```python
from build123d import *

# Parameters (mm, degrees)
SKETCH2_W           = 2.5
SKETCH2_H           = 2.5
BOSS_EXTRUDE1_DEPTH = 39
SKETCH3_W           = 2.5
SKETCH3_H           = 1
BOSS_EXTRUDE2_DEPTH = 3
CUT_EXTRUDE1_DEPTH  = 2.5
FILLET1_R           = 1
BOSS_EXTRUDE3_DEPTH = 2.5
SKETCH8_W           = 2.5
SKETCH8_H           = 2
BOSS_EXTRUDE4_DEPTH = 4


with BuildPart() as part:
    # Sketch2 → Boss-Extrude1 (new body)
    with BuildSketch(Plane(origin=(0, 0, 0), x_dir=(1, 0, 0), z_dir=(0, 1, 0))):
        Rectangle(SKETCH2_W, SKETCH2_H)
    extrude(amount=BOSS_EXTRUDE1_DEPTH)

    # Sketch3 → Boss-Extrude2 (add)
    with BuildSketch(Plane.XY.offset(1.25)):
        with Locations((0, 0.5)):
            Rectangle(SKETCH3_W, SKETCH3_H)
    extrude(amount=BOSS_EXTRUDE2_DEPTH)

    # Sketch4 → Cut-Extrude1 (cut)
    with BuildSketch(Plane(origin=(1.25, 0, 0), x_dir=(0, 0, -1), z_dir=(1, 0, 0))):
        Polygon((-4.25, 0), (-4.25, 0.75), (1.25, 0), align=None)
    extrude(amount=-CUT_EXTRUDE1_DEPTH, mode=Mode.SUBTRACT)

    # Fillet1
    fillet1_edges = [part.edges().sort_by_distance(p)[0] for p in [
        (0, 0, -1.25),
    ]]
    fillet(fillet1_edges, radius=FILLET1_R)

    # Sketch6 → Boss-Extrude3 (add)
    with BuildSketch(Plane.XY.offset(1.25)):
        Polygon((1.25, 20.2), (1.25, 21.8), (3, 21.8), (3, 22.2), (4, 22.2), (4, 19.8), (3, 19.8), (3, 20.2), align=None)
    extrude(amount=-BOSS_EXTRUDE3_DEPTH)

    # Sketch8 → Boss-Extrude4 (add)
    with BuildSketch(Plane.XY.offset(1.25)):
        with Locations((0, 29.4)):
            Rectangle(SKETCH8_W, SKETCH8_H)
    extrude(amount=BOSS_EXTRUDE4_DEPTH)


solid = part.part
```
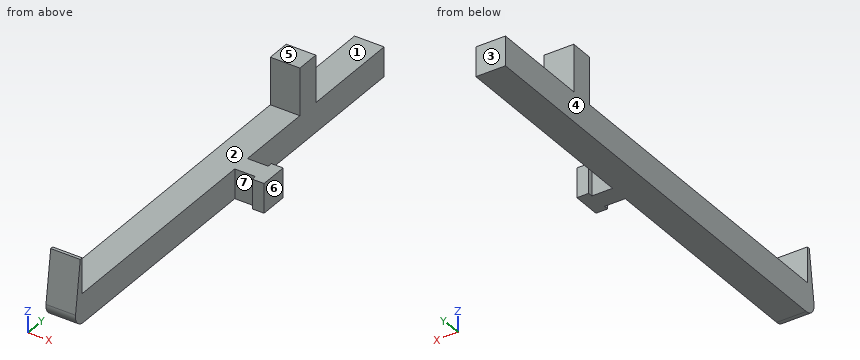
Check sheet for the modelled part. Datum: model origin and axes. Units: mm. Face numbers are marked on the shaded views. A direction names the side the tool comes from. Coordinates: 2 decimals unless noted, no trailing zeros. Write each loop counter-clockwise with the first axis right and the second up, starting at its lowest first coordinate (ties: lowest second). Pieces come first, ordered by that corner, then holes. Notation, with made-up numbers: M 88,41 L 112,41 A27 ccw 112,57 Z; hole C 49,-24 d2. An arc over 180 degrees is marked long. Write item = value, one per line. Start each with the question number.
1. Mould release check, pull along X, two halves, no side actions. Record for the marked faces 4, 5, 6 and 7: pulls with the +X half, pulls with the -X half, needs draft (parallel to the pull), parting line crosses it, or undercut.
2. Sectioned sample at D-D (x = 3.6). Record the cut outline in (y, z).
3. Sectioned sample at C-C (y = 30). Record the cut outline in (x, z).
4. Thickness scan on probe 1 along X at (y, z) = (19.5, 1); probe 2 along Y at (x, z) = (0.85, 4). Record the ranges inside material, lowest first.
5. Go/stop test with flat-tipped pins: pin 1 (2 mm diameter, centred on y = 24, z = 2, fed in from +X); pin 2 (0.8 mm diameter, centred on x = 3.5, z = 0, fed in from +Y); pin 3 (0.5 mm diameter, centred on x = 2, z = 0, fed in from -Y). Record where each tip stops, or that it passes through.
6. Sectioned sample at A-A (x = -0.1). Record the cut outline in (y, z), then the cut area to 3 significant figures.
7. Tool access check on the marked faces 1, 2 and 3. Record the directions out of +Z, -Z, +X, -X, +Y, -Y that give a thin tool (end or side, any length) a straight path to the whole face; none if there is none.
8. Sectioned sample at B-B (z = 0.5). Record the cut outline in (x, y), then the cut area to 3 significant figures.
The answers:
q1.face_4 = pulls with the -X half
q1.face_5 = needs draft
q1.face_6 = pulls with the +X half
q1.face_7 = undercut
q2.outline = M 19.8,-1.25 L 22.2,-1.25 L 22.2,1.25 L 19.8,1.25 Z
q3.outline = M -1.25,-1.25 L 1.25,-1.25 L 1.25,5.25 L -1.25,5.25 Z
q4.probe_1 = -1.25 to 1.25
q4.probe_2 = 0.72 to 1, 28.4 to 30.4
q5.pin_1 = 1.25
q5.pin_2 = 22.2
q5.pin_3 = 20.2
q6.outline = M 0.15,-0.11 A1 ccw 1.15,-1.25 L 39,-1.25 L 39,1.25 L 30.4,1.25 L 30.4,5.25 L 28.4,5.25 L 28.4,1.25 L 1,1.25 L 1,4.25 L 0.75,4.25 Z
q6.area = 106 mm²
q7.face_1 = +Z, +X, -X, +Y
q7.face_2 = +Z, +X, -X
q7.face_3 = +Z, -Z, +X, -X, +Y
q8.outline = M -1.25,0.24 L 1.25,0.24 L 1.25,20.2 L 3,20.2 L 3,19.8 L 4,19.8 L 4,22.2 L 3,22.2 L 3,21.8 L 1.25,21.8 L 1.25,39 L -1.25,39 Z
q8.area = 102 mm²
